Source: CAD feature listing. Evaluate the final solid. Frame: model axes, mm. A direction names the side the tool comes from. Round coordinates to 2 decimals unless told otherwise and drop trailing zeros. Write each loop counter-clockwise with the first axis right and the second up, starting at its lowest first coordinate (ties: lowest second). Pieces come first, ordered by that corner, then holes. Notation, with made-up numbers: M -4.75,72.5 L 13.25,72.5 A11 ccw 13.25,78.5 Z; hole C 10.25,76.25 d4. An arc over 180 degrees is marked long. Put each result on its own line as item: value. Start each with the question number.
Autodesk Fusion 360 part; units mm, degrees
sketch "Sketch1" plane through (0, 0, 0) normal (0, 0, 1) x (1, 0, 0)
  line L0 (0, 0) -> (100, 0)
  line L1 (100, 0) -> (100, 16)
  line L2 (100, 16) -> (0, 16)
  line L3 (0, 16) -> (0, 0)
  line L4 (0, 8) -> (100, 8) construction
  line L5 (50, 16) -> (50, 0) construction
  circle A0 centre (10, 8) radius 2
  circle A1 centre (90, 8) radius 2
  line L6 (19.6419, 16) -> (19.6419, 0)
  line L7 (65, 16) -> (65, 0)
  dimension "d1" = 16
  dimension "d2" = 4
  dimension "d3" = 4
  dimension "d4" = 40
  dimension "d5" = 40
  dimension "d22" = 35
extrude "Extrude1" add sketch "Sketch1" along normal blind 10 contours L0 L2 L3 L6 | L0 L1 L2 L7 makes body 1 at (2.6667, 8, 0) makes body 2 at (72.6667, 8, 0)
extrude "Extrude2" add sketch "Sketch1" along normal blind 5 contours L0 L2 L6 L7 bodies 1 2
fillet "Fillet1" radius 2 1 edges at (0, 8, 10) on bodies 1
fillet "Fillet2" radius 2 1 edges at (100, 8, 10) on bodies 1
fillet "Fillet3" radius 2 3 edges at (0, 16, 4) (0.5858, 16, 9.4142) (10.821, 16, 10) on bodies 1
fillet "Fillet4" radius 2 3 edges at (100, 16, 4) (99.4142, 16, 9.4142) (81.5, 16, 10) on bodies 1
fillet "Fillet5" radius 2 3 edges at (0, 0, 4) (0.5858, 0, 9.4142) (10.821, 0, 10) on bodies 1
fillet "Fillet6" radius 2 3 edges at (81.5, 0, 10) (99.4142, 0, 9.4142) (100, 0, 4) on bodies 1
(1) Access query for faces 1 (the flat face through (19.642, 8, 7)), 2 (the cylindrical face through (99.43, 15.4, 4.06)). Directions: +Z, -Z, +X, -X, +Y, -Y. A direction counts if a zero-diameter tool reaches every point of the face in a straight line with its end or side. Return the directions, or none.
(2) Ray query, line 1 along Y through (x, z) = (90, 4); line 2 along X through (y, z) = (3.75, 8); line 3 along Z through (x, y) = (56, 3.5). Return the intervals inside material, ascending.
(3) Pull-direction query (Y, two-part tool) for faces 3 (the cylindrical face through (10, 6, 5)), 4 (the cylindrical face through (10.94, 15.43, 9.4)), 5 (the flat face through (42, 8, 5)); classes: +Y half, -Y half, draft (parallel to the pull), parting line (faces both ways), or undercut.
(4) Section query D-D (z = 1.5). Return loops of the section in (x, y).
(5) Section query A-A (z = 7). Return loops of the section in (x, y), and give its area (3 significant figures).
(6) Section query B-B (y = 8). Return loops of the section in (x, z).
(7) Section query C-C (x = 90). Return loops of the section in (y, z), and give its area (3 significant figures).
(8) Contact query for a flat-ended pin moving along its axis: P1, Ø8, axis at x = 45.5, y = 5.5, coming from the +Z side. Output: stop coordinate, or through.
Entries:
1. face 1: +Z, +Y, -Y
1. face 2: +Z, -Z, +X, +Y
2. line 1: 0 to 6, 10 to 16
2. line 2: 0 to 19.64, 65 to 100
2. line 3: 0 to 5
3. face 3: undercut
3. face 4: +Y half
3. face 5: draft
4. outline: M 0,2 A2 ccw 2,0 L 98,0 A2 ccw 100,2 L 100,14 A2 ccw 98,16 L 2,16 A2 ccw 0,14 Z; hole C 10,8 d4; hole C 90,8 d4
5. outline: M 0,2 A2 ccw 2,0 L 19.64,0 L 19.64,16 L 2,16 A2 ccw 0,14 Z; M 65,0 L 98,0 A2 ccw 100,2 L 100,14 A2 ccw 98,16 L 65,16 Z; hole C 10,8 d4; hole C 90,8 d4
5. area: 846 mm2
6. outline: M 0,0 L 8,0 L 8,10 L 2,10 A2 ccw 0,8 Z; M 12,0 L 88,0 L 88,10 L 65,10 L 65,5 L 19.64,5 L 19.64,10 L 12,10 Z; M 92,0 L 100,0 L 100,8 A2 ccw 98,10 L 92,10 Z
7. outline: M 0,0 L 6,0 L 6,10 L 2,10 A2 ccw 0,8 Z; M 10,0 L 16,0 L 16,8 A2 ccw 14,10 L 10,10 Z
7. area: 118 mm2
8. P1: z = 5
